The listing builds one solid part. Answer for the finished solid, in the listing's coordinates (mm). Give positions to 0.01 mm unless a question says otherwise; leave off trailing zeros. Write each loop counter-clockwise with the first axis right and the second up, starting at its lowest first coordinate (ties: lowest second). Pieces come first, ordered by that corner, then holes. Notation, with made-up numbers: (37.5, 2.25) - (64.5, 2.25) arc R10 ccw to (64.5, 14.25) - close; hole circle Ø5 at (48, 55.5). An arc over 180 degrees is marked (long way). Use a Markdown table: item, result. Add a question column.
Autodesk Inventor part; units mm, degrees
ref_plane "YZ Plane" through (0, 0, 0) normal (1, 0, 0) x (0, 1, 0)
ref_plane "XZ Plane" through (0, 0, 0) normal (0, 1, 0) x (-1, 0, 0)
ref_plane "XY Plane" through (0, 0, 0) normal (0, 0, 1) x (1, 0, 0)
sketch "Boceto1" plane through (0, 0, 0) normal (1, 0, 0) x (0, 1, 0)
  line L0 (-80, -110) -> (80, -110)
  line L1 (80, -110) -> (80, 110)
  line L2 (80, 110) -> (-80, 110)
  line L3 (-80, 110) -> (-80, -110)
  line L4 (-80, -110) -> (80, 110) construction
  line L5 (80, -110) -> (-80, 110) construction
  point P0 (0, 0)
  dimension "d0" = 160
  dimension "d1" = 220
extrude "Extrusión1" add sketch "Boceto1" along normal blind 10
sketch "Boceto2" plane through (0, 0, 0) normal (-1, 0, 0) x (0, 0, 1)
  line L0 (-110, 80) -> (110, 80)
  line L1 (110, 80) -> (110, -80)
  line L2 (-110, -80) -> (-110, 80)
  line L3 (-110, -80) -> (-110, 80) construction
  line L4 (-110, 0) -> (110, 0) construction
  point P0 (0, 0)
  point P1 (0, -75)
  point P2 (-80, -75)
  point P3 (80, -75)
hole "Agujero1" at (0, -75, -80) at (0, -75, 0) at (0, -75, 80) direction (1, 0, 0) diameter 5.5 depth 20 tip angle 118 countersink diameter 11 countersink angle 90
properties part number "LATERAL B" material "Plástico PMMA"
1. For a pull along Z with two mould halves and no side action, classify faces 1 (the cylindrical face through (6.426, -75.121, 77.253)), 2 (the flat face through (5, -1, -110)), 3 (the flat face through (5, -80, 2)) as released by +Z, released by -Z, zero draft, split by the parting line, or undercut.
2. The part is cut by section A-A (y = -75). Give the vertices of the cut face in (x, z), and give its area (3 significant figures).
3. Consider L1, parallel to Z at x = 8.25, y = -75; L2, parallel to Y at x = 6, z = 80; L3, parallel to Z at x = 7.75, y = -72.5. Determine where each line is inside the solid, lowest interval first. Write a range as [from, to].
4. Given P1, Ø6.5, axis at y = -75, z = 0, coming from the -X side, flat-ended and moving along its own axis, determine where the tip first touches the part or whether it passes through.
5. The part is cut by section B-B (z = 80). Give the vertices of the cut face in (x, y).
Check values:
| question | item | result |
|---|---|---|
| 1 | face 1 | undercut |
| 1 | face 2 | released by -Z |
| 1 | face 3 | zero draft |
| 2 | outline | (0, -110) - (10, -110) - (10, -82.75) - (2.75, -82.75) - (0, -85.5) - close; (0, -74.5) - (2.75, -77.25) - (10, -77.25) - (10, -2.75) - (2.75, -2.75) - (0, -5.5) - close; (0, 5.5) - (2.75, 2.75) - (10, 2.75) - (10, 77.25) - (2.75, 77.25) - (0, 74.5) - close; (0, 85.5) - (2.75, 82.75) - (10, 82.75) - (10, 110) - (0, 110) - close |
| 2 | area | 2,010 mm2 |
| 3 | L1 | z = [-110, -82.75], [-77.25, -2.75], [2.75, 77.25], [82.75, 110] |
| 3 | L2 | y = [-80, -77.75], [-72.25, 80] |
| 3 | L3 | z = [-110, -81.15], [-78.85, -1.15], [1.15, 78.85], [81.15, 110] |
| 4 | P1 | stops at x = 2.25 |
| 5 | outline | (0, -69.5) - (2.75, -72.25) - (10, -72.25) - (10, 80) - (0, 80) - close; (0.5, -80) - (10, -80) - (10, -77.75) - (2.75, -77.75) - close |
